from build123d import *

# Parameters (mm, degrees)
F0_R     = 4.826
F0_R_2   = 2.5527
F0_R_3   = 4.7625
F0_R_4   = 3.175
F0_R_5   = 14.28115
F1_DEPTH = 12


with BuildPart() as f1:
    # F0 (on Front) → F1 (new body)
    with BuildSketch(Plane.XZ):
        with BuildLine():
            Line((-423.736694, 132.242903), (-584.775201, 80.589762))
            ThreePointArc((-584.775201, 80.589762), (-600.913731, 48.498208), (-568.822177, 32.359678))
            Line((-568.822177, 32.359678), (-392.250095, 92.377704))
            Line((-392.250095, 92.377704), (-212.8567, 234.067401))
            ThreePointArc((-212.8567, 234.067401), (-208.667401, 269.7433), (-244.3433, 273.932599))
            Line((-244.3433, 273.932599), (-264.275899, 258.1893))
            Line((-264.275899, 258.1893), (-311.505798, 317.987098))
            ThreePointArc((-311.505798, 317.987098), (-347.181697, 322.176398), (-351.370997, 286.500499))
            Line((-351.370997, 286.500499), (-304.141098, 226.702701))
            Line((-304.141098, 226.702701), (-423.736694, 132.242903))
        make_face()
        with Locations((-576.798689, 56.47472)):
            Circle(F0_R, mode=Mode.SUBTRACT)
        with Locations((-552.683647, 64.451232)):
            Circle(F0_R_2, mode=Mode.SUBTRACT)
        with Locations((-528.568605, 72.427744)):
            Circle(F0_R_2, mode=Mode.SUBTRACT)
        with Locations((-504.453563, 80.404256)):
            Circle(F0_R_2, mode=Mode.SUBTRACT)
        with Locations((-480.338521, 88.380768)):
            Circle(F0_R_2, mode=Mode.SUBTRACT)
        with Locations((-456.223479, 96.35728)):
            Circle(F0_R_2, mode=Mode.SUBTRACT)
        with Locations((-432.108436, 104.333792)):
            Circle(F0_R_2, mode=Mode.SUBTRACT)
        with Locations((-407.993394, 112.310304)):
            Circle(F0_R_3, mode=Mode.SUBTRACT)
        with Locations((-388.060795, 128.053603)):
            Circle(F0_R_2, mode=Mode.SUBTRACT)
        with Locations((-368.128196, 143.796903)):
            Circle(F0_R_2, mode=Mode.SUBTRACT)
        with Locations((-348.195596, 159.540202)):
            Circle(F0_R_2, mode=Mode.SUBTRACT)
        with Locations((-328.262997, 175.283502)):
            Circle(F0_R_2, mode=Mode.SUBTRACT)
        with Locations((-308.330397, 191.026802)):
            Circle(F0_R_2, mode=Mode.SUBTRACT)
        with Locations((-288.397798, 206.770101)):
            Circle(F0_R_2, mode=Mode.SUBTRACT)
        with Locations((-297.941588, 231.599239)):
            Circle(F0_R_2, mode=Mode.SUBTRACT)
        with Locations((-268.465199, 222.513401)):
            Circle(F0_R_2, mode=Mode.SUBTRACT)
        with Locations((-270.475408, 253.292762)):
            Circle(F0_R_2, mode=Mode.SUBTRACT)
        with Locations((-248.532599, 238.2567)):
            Circle(F0_R_2, mode=Mode.SUBTRACT)
        with Locations((-317.246, 255.27)):
            Circle(F0_R_2, mode=Mode.SUBTRACT)
        with Locations((-336.550412, 278.940761)):
            Circle(F0_R_2, mode=Mode.SUBTRACT)
        with Locations((-331.438397, 302.243798)):
            Circle(F0_R_4, mode=Mode.SUBTRACT)
        with Locations((-309.084231, 300.634284)):
            Circle(F0_R_2, mode=Mode.SUBTRACT)
        with Locations((-289.77982, 276.963523)):
            Circle(F0_R_2, mode=Mode.SUBTRACT)
        with Locations((-228.6, 254)):
            Circle(F0_R_5, mode=Mode.SUBTRACT)
    extrude(amount=F1_DEPTH)


solid = f1.part
For this review, take the finished solid that the model builds, in its own axes (mm). A direction names the side the tool comes from. Give positions to 0.01 mm unless a question says otherwise; leave off trailing zeros. Loops run counter-clockwise (first coordinate to the right, second up) from the corner with the lowest first, then second, coordinate; pieces in that order, holes last.
Item 1: For line 1 along X through (y, z) = (-6.75, 255.27); line 2 along X through (y, z) = (-4.5, 265.5); line 3 along X through (y, z) = (-6.5, 275.5), list the stretches that pass through material, from the lowest coordinate up.
Item 2: Take a section at C-C, the plane z = 167. State the section outline as (x, y) points.
Item 3: Take a section at A-A, the plane x = -228.6. State the section outline as (y, z) points, and give its area (3 significant figures).
Item 4: Draft analysis for pull direction X (two halves, no side actions). For faces 1 (the flat face through (-328.087, -5.916, 257.02)), 2 (the flat face through (-303.81, -5.92, 162.23)), 3 (the cylindrical face through (-581.62, -5.92, 56.69)), 4 (the flat face through (-389, 0, 158)), state which applies: +X half, -X half, draft (parallel to the pull), parting line (faces both ways), or undercut.
Item 5: Take a section at B-B, the plane z = 121.5. State the section outline as (x, y) points, and give its area (3 significant figures).
Item 6: Tool access review of faces 5 (the flat face through (-363.102, -5.916, 180.134)), 6 (the flat face through (-287.56, -5.92, 287.67)), 7 (the flat face through (-389, -12, 158)): name each direction out of +Z, -Z, +X, -X, +Y, -Y from which nothing blocks a thin tool from reaching the whole face with its end or side.
Item 7: Insertion check: pin 1 (1 mm diameter, centred on x = -518.5, y = -6, fed in from -Z); pin 2 (3 mm diameter, centred on y = -3.5, z = 101, fed in from +X); pin 3 (5 mm diameter, centred on x = -272, y = -2, fed in from +Z). Each pin has a flat end and moves straight along its axis. Give the tip position at first contact, or say it passes through.
Calculated:
1. line 1: x = -326.7 to -319.8, -314.69 to -272.09, -268.86 to -242.82, -214.38 to -203.23
1. line 2: x = -334.78 to -270.05, -255.02 to -237.07, -220.13 to -205.95
1. line 3: x = -342.68 to -291.87, -287.69 to -277.95, -242.12 to -215.08
2. outline: (-379.73, -12) - (-297.77, -12) - (-297.77, 0) - (-379.73, 0) - close
3. outline: (-12, 221.63) - (0, 221.63) - (0, 239.72) - (-12, 239.72) - close; (-12, 268.28) - (0, 268.28) - (0, 279.4) - (-12, 279.4) - close
3. area: 350 mm2
4. face 1: -X half
4. face 2: +X half
4. face 3: undercut
4. face 4: draft
5. outline: (-457.23, -12) - (-355.38, -12) - (-355.38, 0) - (-457.23, 0) - close
5. area: 1,220 mm2
6. face 5: -X, +Y, -Y
6. face 6: +Z, +Y, -Y
6. face 7: +Z, -Z, +X, -X, -Y
7. pin 1: stops at z = 49.29
7. pin 2: stops at x = -379.43
7. pin 3: stops at z = 271.13
